from build123d import *

# Parameters (mm, degrees)
F2_R           = 4.7625
F2_R_2         = 2.5
F3_DEPTH       = 7.501
F5_D           = 5
F5_CSINK_D     = 10
F5_CSINK_ANGLE = 90


with BuildPart() as f1:
    # F0 (on Front) → F1 (revolve)
    with BuildSketch(Plane.XZ):
        with BuildLine():
            Line((0, 19), (0, 0))
            Line((0, 0), (4, 0))
            Line((4, 0), (4, 9))
            Line((4, 9), (7.5, 9))
            Line((7.5, 9), (7.5, 19))
            Line((7.5, 19), (6.13125, 19))
            Line((6.13125, 19), (6.13125, 15.08125))
            ThreePointArc((6.13125, 15.08125), (3.75, 12.7), (1.36875, 15.08125))
            Line((1.36875, 15.08125), (1.36875, 19))
            Line((1.36875, 19), (0, 19))
        make_face()
    revolve(axis=Axis((2, 0, 0), (-1, 0, 0)))

    # F2 (on face) → F3 (cut, through all)
    with BuildSketch(Plane.YZ.offset(7.5)):
        Circle(F2_R)
        with Locations((0, 9.525)):
            Circle(F2_R_2)
        with Locations((9.525, 0)):
            Circle(F2_R_2)
        with Locations((0, -9.525)):
            Circle(F2_R_2)
        with Locations((-9.525, 0)):
            Circle(F2_R_2)
    extrude(amount=-F3_DEPTH, mode=Mode.SUBTRACT)

    # F5 (through all)
    with Locations(Plane(origin=(0, 0, 0), x_dir=(0, -1, 0), z_dir=(-1, 0, 0))):
        with Locations((0, 9.525), (9.525, 0), (0, -9.525), (-9.525, 0)):
            CounterSinkHole(F5_D / 2, F5_CSINK_D / 2, counter_sink_angle=F5_CSINK_ANGLE)


solid = f1.part
Design review of the part built by this model. Coordinates are the model's own, in mm. A direction names the side the tool comes from. Round coordinates to 2 decimals unless told otherwise and drop trailing zeros.
1) Clearance check with flat-ended pins moving along their axes: pin 1 Ø14 at (y, z) = (1.5, -1) entering from +X; pin 2 Ø2 at (x, z) = (3, -4) entering from +Y; pin 3 Ø6.5 at (y, z) = (0, -9.525) entering from -X. State where each tip first meets the part, or that it passes through.
The answers:
pin 1: stops at x = 4
pin 2: stops at y = 12.9
pin 3: stops at x = 1.75
2) Consider section A-A (y = 0). Count the separate pieces of the cut face and the enclosed holes in it, plus the area to 3 significant figures.
The answers:
separate pieces: 4
enclosed holes: 0
area: 55.1 mm2
3) Machinability: for faces 4 (the cylindrical face through (5.035, 1.154, -11.743)), 5 (the cylindrical face through (5.77, -6.41, 6.32)), 6 (the flat face through (1.369, 14, 6)), which of the approach directions +Z, -Z, +X, -X, +Y, -Y give a long, thin tool a straight path to every point of the face, cutting with its end or side? Answer none if there is none.
The answers:
face 4: +X, -X
face 5: +X
face 6: none
4) For L1, parallel to Y at x = 6.5, z = 0 (3 decimals); L2, parallel to Z at x = 1, y = -2; L3, parallel to X at y = 11, z = 12, list the stretches that pass through material, from the lowest coordinate up.
The answers:
L1: y = -19 to -12.025, 12.025 to 19
L2: z = -18.89 to -12.99, -6.06 to -4.32, 4.32 to 6.06, 12.99 to 18.89
L3: x = 0 to 1.37, 6.13 to 7.5
5) Draft analysis for pull direction Y (two halves, no side actions). For faces 1 (the cylindrical face through (6.806, -16.856, 8.767)), 2 (the flat face through (6.131, 14, -6)), 3 (the conical face through (2.38, -0.34, -6.93)), state which applies: released by +Y, released by -Y, zero draft, split by the parting line, or undercut.
The answers:
face 1: split by the parting line
face 2: zero draft
face 3: undercut
